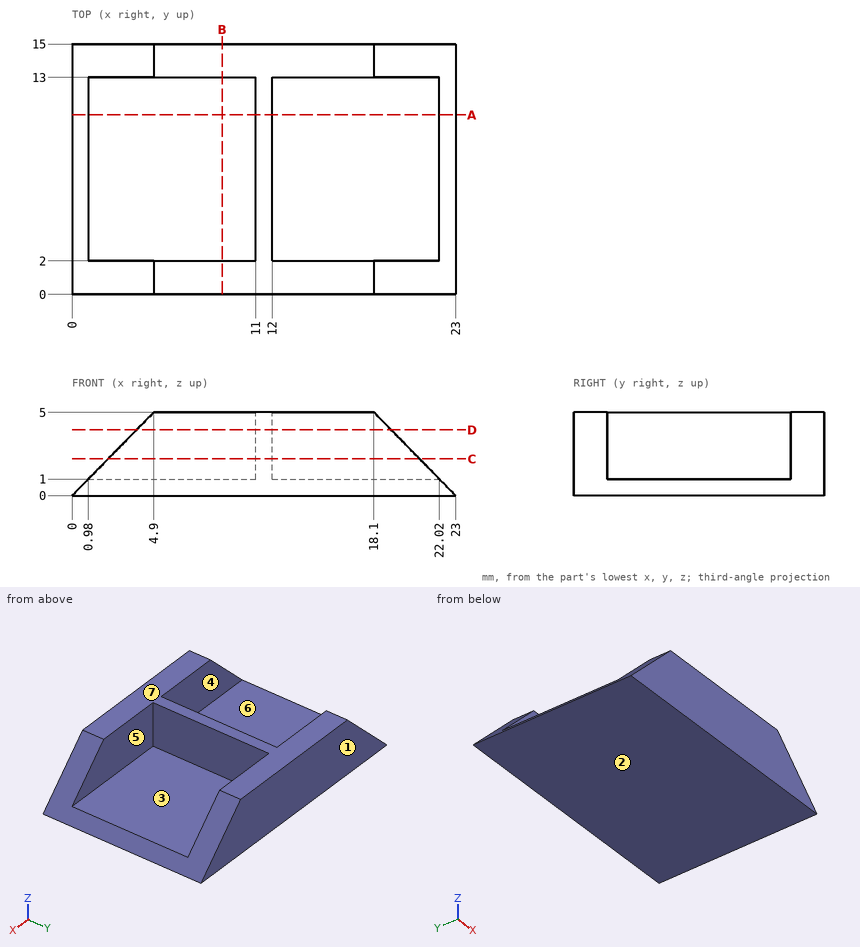
Source: three-view drawing plus pictorial views. Frame: mm from the lowest corner of the part. A direction names the side the tool comes from. Coordinates: 2 decimals unless noted, no trailing zeros. Loops run counter-clockwise (first coordinate to the right, second up) from the corner with the lowest first, then second, coordinate; pieces in that order, holes last. Notation, with made-up numbers: (23.5, -10.75) -> (68.5, -10.75) arc R23 ccw to (68.5, 4.25) -> close; hole circle Ø2 at (-22, 12). An arc over 180 degrees is marked (long way). One line per item, written item: value.
(1) Pin query (flat end, axial travel): pin 1 Ø8 at (x, y) = (19, 7.5) entering from +Z; pin 2 Ø1 at (y, z) = (9.5, 3.5) entering from -X; pin 3 Ø2 at (y, z) = (7.5, 3) entering from +X. Return the tip coordinate at first contact, or that it passes through.
Answer below:
pin 1: stops at z = 1
pin 2: stops at x = 11
pin 3: stops at x = 12
(2) Cut plane D-D (z = 3.95). Output: boundary loops of the cut face in (x, y).
Answer below:
outline: (3.87, 0) -> (19.13, 0) -> (19.13, 2) -> (12, 2) -> (12, 13) -> (19.13, 13) -> (19.13, 15) -> (3.87, 15) -> (3.87, 13) -> (11, 13) -> (11, 2) -> (3.87, 2) -> close
(3) Cut plane A-A (y = 10.75). Output: boundary loops of the cut face in (x, z).
Answer below:
outline: (0, 0) -> (23, 0) -> (22.02, 1) -> (12, 1) -> (12, 5) -> (11, 5) -> (11, 1) -> (0.98, 1) -> close
(4) Set-up query: the marked faces 5, 6 and 7. Return all of +Z, -Z, +X, -X, +Y, -Y with unobstructed straight access to the full face (end or side cutting, diameter ignored); none if empty.
Answer below:
face 5: +Z, +X
face 6: +Z, -X
face 7: +Z, +X, -X, +Y, -Y
(5) Cut plane C-C (z = 2.2). Output: boundary loops of the cut face in (x, y).
Answer below:
outline: (2.16, 0) -> (20.84, 0) -> (20.84, 2) -> (12, 2) -> (12, 13) -> (20.84, 13) -> (20.84, 15) -> (2.16, 15) -> (2.16, 13) -> (11, 13) -> (11, 2) -> (2.16, 2) -> close
(6) Ray query, line 1 along Y through (x, z) = (4, 1.3); line 2 along Z through (x, y) = (16.5, 9); line 3 along X through (y, z) = (8.25, 4.6). Return the intervals inside material, ascending.
Answer below:
line 1: y = 0 to 2, 13 to 15
line 2: z = 0 to 1
line 3: x = 11 to 12
(7) Cut plane B-B (x = 9). Output: boundary loops of the cut face in (y, z).
Answer below:
outline: (0, 0) -> (15, 0) -> (15, 5) -> (13, 5) -> (13, 1) -> (2, 1) -> (2, 5) -> (0, 5) -> close
(8) Draft query along Y for the marked faces 1, 2, 3 and 4. Return one class per face: pulls with the +Y half, pulls with the -Y half, needs draft (parallel to the pull), parting line crosses it, or undercut.
Answer below:
face 1: pulls with the +Y half
face 2: needs draft
face 3: undercut
face 4: undercut
